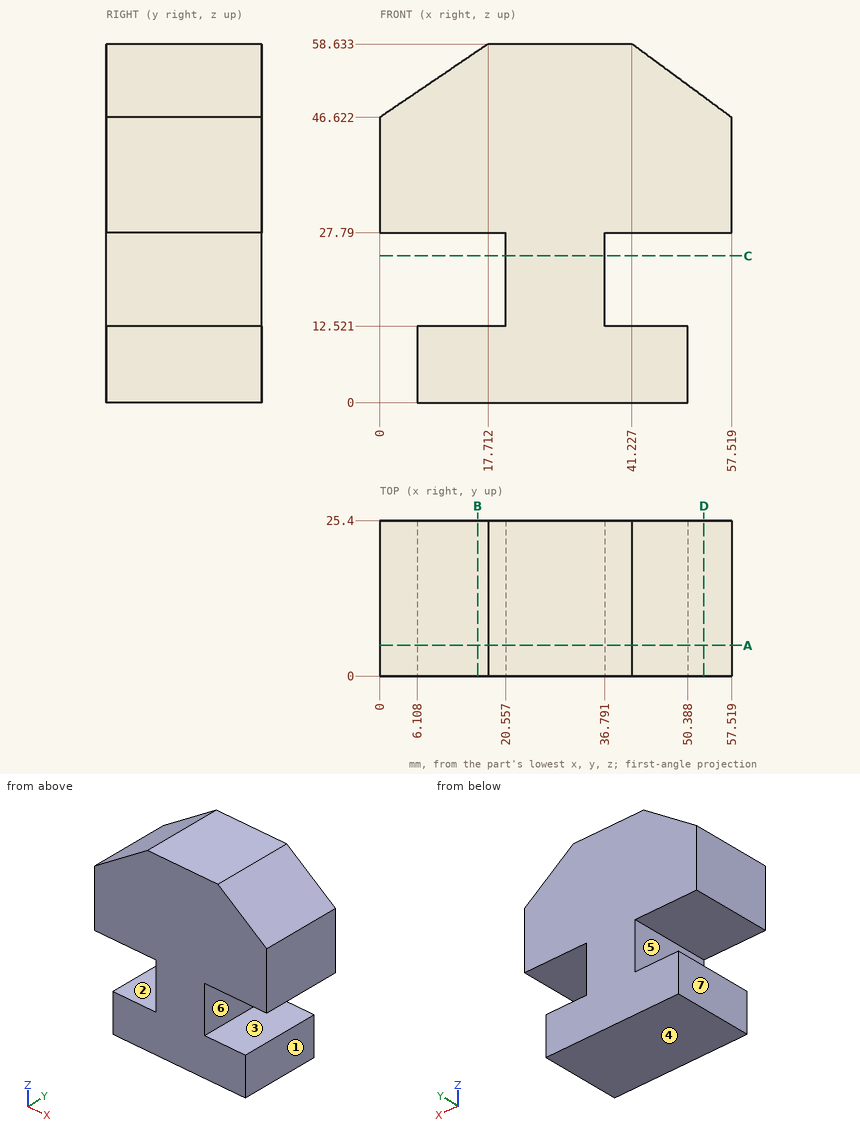
Print and shaded views of the part. All mm, measured from the part's lowest x, y and z. A direction names the side the tool comes from. Give positions to 0.01 mm unless a question says otherwise; leave off trailing zeros. Write each loop counter-clockwise with the first axis right and the second up, starting at its lowest first coordinate (ties: lowest second). Pieces come first, ordered by that corner, then holes. Notation, with made-up numbers: M 27,5 L 70,5 A24 ccw 70,32 Z; hole C 75,51.5 d3. An arc over 180 degrees is marked long. Use a Markdown table: item, result.
1) Drill centre lines: line 1 (Z direction, x = 39, y = 18.75); line 2 (X direction, y = 7.25, z = 16); line 3 (Z direction, x = 14, y = 21.5) (1 decimal). Where is each one in solid material? Low to high. Write a range as from..to.
Responses:
| item | result |
|---|---|
| line 1 | z = 0..12.52, 27.79..58.63 |
| line 2 | x = 20.56..36.79 |
| line 3 | z = 0..12.5, 27.8..56.1 |
2) Tool access for the marked faces 1, 2 and 3: list every direction of +Z, -Z, +X, -X, +Y, -Y with a clear straight run to the whole face (end or side of a thin tool).
Responses:
| item | result |
|---|---|
| face 1 | -Z, +X, +Y, -Y |
| face 2 | -X, +Y, -Y |
| face 3 | +X, +Y, -Y |
3) Cut at B-B (x = 16). List the corners of the cut face in (y, z), and give its area (3 significant figures).
Responses:
| item | result |
|---|---|
| outline | M 0,0 L 25.4,0 L 25.4,12.52 L 0,12.52 Z; M 0,27.79 L 25.4,27.79 L 25.4,57.47 L 0,57.47 Z |
| area | 1,070 mm2 |
4) Cut at C-C (z = 24). List the corners of the cut face in (x, y).
Responses:
| item | result |
|---|---|
| outline | M 20.56,0 L 36.79,0 L 36.79,25.4 L 20.56,25.4 Z |
5) Pin check, flat tips, straight feed: pin 1 (12 mm diameter, centred on y = 15.5, z = 19.5, fed in from +X); pin 2 (14 mm diameter, centred on y = 6.5, z = 5, fed in from +X); pin 3 (1 mm diameter, centred on x = 42.5, y = 18, fed in from +Z). Stop position of each tip, or through.
Responses:
| item | result |
|---|---|
| pin 1 | stops at x = 36.79 |
| pin 2 | stops at x = 50.39 |
| pin 3 | stops at z = 58.06 |
6) Cut at A-A (y = 5). List the corners of the cut face in (x, z).
Responses:
| item | result |
|---|---|
| outline | M 0,27.79 L 20.56,27.79 L 20.56,12.52 L 6.11,12.52 L 6.11,0 L 50.39,0 L 50.39,12.52 L 36.79,12.52 L 36.79,27.79 L 57.52,27.79 L 57.52,46.62 L 41.23,58.63 L 17.71,58.63 L 0,46.62 Z |
7) Cut at D-D (x = 53). List the corners of the cut face in (y, z), and give its area (3 significant figures).
Responses:
| item | result |
|---|---|
| outline | M 0,27.79 L 25.4,27.79 L 25.4,49.95 L 0,49.95 Z |
| area | 563 mm2 |
8) Pull direction Z, two halves, no side cores. Call the marked faces 4, 5, 6 and 7: +Z half, -Z half, draft (parallel to the pull), parting line (faces both ways), or undercut.
Responses:
| item | result |
|---|---|
| face 4 | -Z half |
| face 5 | undercut |
| face 6 | undercut |
| face 7 | draft |
